from build123d import *

# Parameters (mm, degrees)
SKETCH_2_R          = 3
EXTRUDE_1_DEPTH     = 3
CUT_EXTRUDE_1_DEPTH = 28.407077077
FILLET_1_R          = 14


with BuildPart() as part:
    # 草图2 → 凸台-拉伸1 (new body)
    with BuildSketch(Plane(origin=(0, 0, 0), x_dir=(1, 0, 0), z_dir=(0, 1, 0))):
        with BuildLine():
            ThreePointArc((2.5, -2.449489743), (0, 3.5), (-2.5, -2.449489743))
            Line((-2.5, -2.449489743), (-2.5, -17.449489743))
            ThreePointArc((-2.5, -17.449489743), (0, -26.779616762), (2.5, -17.449489743))
            Line((2.5, -17.449489743), (2.5, -2.449489743))
        make_face()
        with BuildLine():
            Line((1, 1.118033989), (1, -1.118033989))
            ThreePointArc((1, -1.118033989), (-1.5, 0), (1, 1.118033989))
        make_face(mode=Mode.SUBTRACT)
        with Locations(Location((0, -21.779616762, 0), (0, 0, 270))):
            Circle(SKETCH_2_R, mode=Mode.SUBTRACT)
    extrude(amount=EXTRUDE_1_DEPTH)

    # 草图3 → 切除-拉伸1 (cut, through all)
    with BuildSketch(Plane.XZ):
        with BuildLine():
            ThreePointArc((2.5, 17.449489743), (2.253537793, 17.31625845), (2, 17.197041067))
            Line((2, 17.197041067), (2, 2.872281323))
            ThreePointArc((2, 2.872281323), (2.259908888, 2.67260394), (2.5, 2.449489743))
            Line((2.5, 2.449489743), (2.5, 17.449489743))
        make_face()
    extrude(amount=-CUT_EXTRUDE_1_DEPTH, mode=Mode.SUBTRACT)

    # 圆角1
    fillet_1_edges = [part.edges().sort_by_distance(p)[0] for p in [
        (2, 1.5, 2.872281323),
        (2, 1.5, 17.197041067),
    ]]
    fillet(fillet_1_edges, radius=FILLET_1_R)


solid = part.part
Build history of the part. All positions in model axes, mm. A direction names the side the tool comes from. Give positions to 0.01 mm unless a question says otherwise; leave off trailing zeros. Loops run counter-clockwise (first coordinate to the right, second up) from the corner with the lowest first, then second, coordinate; pieces in that order, holes last. Notation, with made-up numbers: (30.25, 55.25) - (37.25, 55.25) arc R22 ccw to (37.25, 77.25) - close; hole circle Ø8 at (76, 25.25). An arc over 180 degrees is marked (long way). Write item = value, one per line. Start each with the question number.
1) Band-saw the part on C-C on y = 2.6. Count the separate pieces of the cut face and the enclosed holes in it, plus the area to 3 significant figures.
2) Pull direction X, two halves, no side cores. Call faces 4 (the flat face through (-2.5, 1, 10)), 5 (the cylindrical face through (-1.5, 1.5, 0)), 6 (the cylindrical face through (-1.344, 1.479, 26.596)): +X half, -X half, draft (parallel to the pull), parting line (faces both ways), or undercut.
3) Band-saw the part on B-B on z = 0. Give the cut face in (x, y), plus the area to 3 significant figures.
4) Probe probe 1 along Z at (x, y) = (-0.25, 2.5); probe 2 along Z at (x, y) = (-2.75, 1.8); probe 3 along X at (y, z) = (0.35, 23.5). List the from-to ranges inside material, lowest first. Write a range as from..to.
5) Drop flat-ended pins along their axis: pin 1 Ø1.8 at (y, z) = (2, 0.5) entering from -X; pin 2 Ø0.9 at (y, z) = (1.5, 9.5) entering from +X; pin 3 Ø1.5 at (y, z) = (1.5, 5.5) entering from -X; pin 4 Ø5.5 at (x, z) = (0, 21.78) entering from +Y. Give the stop position or say it passes through.
6) Band-saw the part on A-A on x = 0. Give the cut face in (y, z), plus the area to 3 significant figures.
7) Tool access for faces 1 (the flat face through (0, 3, 11)), 2 (the flat face through (1, 1, 0)), 3 (the flat face through (2, 1, 9)): list every direction of +Z, -Z, +X, -X, +Y, -Y with a clear straight run to the whole face (end or side of a thin tool).
Final values:
q1.separate_pieces = 1
q1.enclosed_holes = 2
q1.area = 148 mm²
q2.face_4 = -X half
q2.face_5 = undercut
q2.face_6 = parting line
q3.outline = (-3.5, 0) - (-1.5, 0) - (-1.5, 3) - (-3.5, 3) - close; (1, 0) - (3.5, 0) - (3.5, 3) - (1, 3) - close
q3.area = 13.5 mm²
q4.probe_1 = -3.49..-1.48, 1.48..18.79, 24.77..26.77
q4.probe_2 = -2.17..2.17, 17.6..20.58, 22.98..25.96
q4.probe_3 = -4.69..-2.46, 2.46..4.69
q5.pin_1 = -3.5
q5.pin_2 = 2
q5.pin_3 = -2.5
q5.pin_4 = through
q6.outline = (0, -3.5) - (3, -3.5) - (3, -1.5) - (0, -1.5) - close; (0, 1.5) - (3, 1.5) - (3, 18.78) - (0, 18.78) - close; (0, 24.78) - (3, 24.78) - (3, 26.78) - (0, 26.78) - close
q6.area = 63.8 mm²
q7.face_1 = +Z, -Z, +X, -X, +Y
q7.face_2 = +Y, -Y
q7.face_3 = +X, +Y, -Y
